Build history of the part. All positions in model axes, mm. Face numbers are marked on the shaded views. A direction names the side the tool comes from. Round coordinates to 2 decimals unless told otherwise and drop trailing zeros. Order: outer loops, then holes, each group sorted by start corner. A loop starts at its lowest first (then second) coordinate and runs counter-clockwise, first axis right, second up. Notation, with made-up numbers: M 70,37 L 109,37 A19 cw 109,57 Z; hole C 66.25,-27 d8. An arc over 180 degrees is marked long. One line per item, written item: value. Start each with the question number.
Item 1: Pin check, flat tips, straight feed: pin 1 (4 mm diameter, centred on y = 52, z = 318.5, fed in from -X); pin 2 (17 mm diameter, centred on x = -101.5, y = 0, fed in from +Z); pin 3 (3 mm diameter, centred on y = 176.5, z = 327, fed in from -X). Stop position of each tip, or through.
Item 2: Band-saw the part on B-B, the plane y = 56.5. Write the cut outline in (x, z).
Item 3: Band-saw the part on C-C, the plane z = 386. Write the cut outline in (x, y).
Item 4: Tool access for the marked faces 1, 2 and 3: list every direction of +Z, -Z, +X, -X, +Y, -Y with a clear straight run to the whole face (end or side of a thin tool).
Item 5: Band-saw the part on A-A, the plane z = 174.5. Write the cut outline in (x, y), then the cut area to 3 significant figures.
Item 6: Band-saw the part on D-D, the plane x = -101.5. Write the cut outline in (y, z).
Item 7: Probe L1, parallel to X at y = 205, z = 174.5; L2, parallel to Y at x = 101.5, z = 150.5; L3, parallel to Y at x = 77.5, z = 200.5. List the from-to ranges inside material, lowest first.
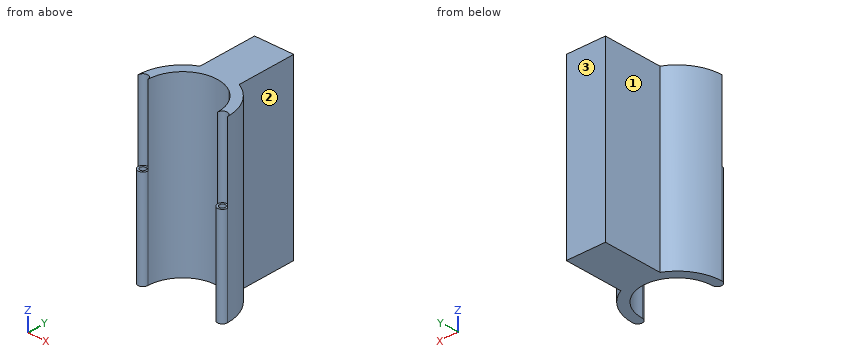
```python
from build123d import *

# Parameters (mm, degrees)
BOSS_EXTRU_1_DEPTH      = 450
ESQUISSE2_R             = 7.5
ENL_V_MAT_EXTRU_1_DEPTH = 350
ESQUISSE2_3_R           = 12.5
ESQUISSE2_3_R_2         = 7.5
ENL_V_MAT_EXTRU_2_DEPTH = 200


with BuildPart() as part:
    # Esquisse1 → Boss.-Extru.1 (new body)
    with BuildSketch(Plane.XY):
        with BuildLine():
            Line((-50, 253.627440537), (-50, 102.449987799))
            ThreePointArc((-50, 102.449987799), (0, 114), (50, 102.449987799))
            Line((50, 102.449987799), (50, 253.627440537))
            Line((50, 253.627440537), (-50, 253.627440537))
        make_face()
        with BuildLine():
            ThreePointArc((-89, 0), (-78.647949751, 41.659332688), (-50, 73.627440537))
            Line((-50, 73.627440537), (-50, 102.449987799))
            ThreePointArc((-50, 102.449987799), (-96.685055722, 60.398675482), (-114, 0))
            ThreePointArc((-114, 0), (-101.5, -12.5), (-89, 0))
        make_face()
        with BuildLine():
            Line((-50, 102.449987799), (-50, 73.627440537))
            ThreePointArc((-50, 73.627440537), (0, 89), (50, 73.627440537))
            Line((50, 73.627440537), (50, 102.449987799))
            ThreePointArc((50, 102.449987799), (0, 114), (-50, 102.449987799))
        make_face()
        with BuildLine():
            Line((50, 102.449987799), (50, 73.627440537))
            ThreePointArc((50, 73.627440537), (78.647949751, 41.659332688), (89, 0))
            ThreePointArc((89, 0), (101.5, -12.5), (114, 0))
            ThreePointArc((114, 0), (96.685055722, 60.398675482), (50, 102.449987799))
        make_face()
    extrude(amount=BOSS_EXTRU_1_DEPTH)

    # Esquisse2 → Enl_v. mat.-Extru.1 (cut)
    with BuildSketch(Plane.XY.offset(450)):
        with Locations((101.5, 0)):
            Circle(ESQUISSE2_R)
        with Locations((-101.5, 0)):
            Circle(ESQUISSE2_R)
    extrude(amount=-ENL_V_MAT_EXTRU_1_DEPTH, mode=Mode.SUBTRACT)

    # Esquisse2_3 → Enl_v. mat.-Extru.2 (cut)
    # profile 1 of 2: a face of its own
    with BuildSketch(Plane.XY.offset(450)):
        with Locations((-101.5, 0)):
            Circle(ESQUISSE2_3_R)
        with Locations((-101.5, 0)):
            Circle(ESQUISSE2_3_R_2, mode=Mode.SUBTRACT)
    # profile 2 of 2: a face of its own
    with BuildSketch(Plane.XY.offset(450)):
        with Locations((101.5, 0)):
            Circle(ESQUISSE2_3_R)
        with Locations((101.5, 0)):
            Circle(ESQUISSE2_3_R_2, mode=Mode.SUBTRACT)
    extrude(amount=-ENL_V_MAT_EXTRU_2_DEPTH, mode=Mode.SUBTRACT)


solid = part.part
```
Output:
1. pin 1: stops at x = -102.45
1. pin 2: stops at z = 250
1. pin 3: stops at x = -50
2. outline: M -99.01,0 L -68.77,0 L -68.77,450 L -99.01,450 Z; M 68.77,0 L 99.01,0 L 99.01,450 L 68.77,450 Z
3. outline: M -114,0 A12.5 cw -89,0 A89 cw 89,0 A12.5 cw 114,0 A114 ccw 50,102.45 L 50,253.63 L -50,253.63 L -50,102.45 A114 ccw Z
4. face 1: +Z, -Z, -X, +Y
4. face 2: +Z, -Z, +X, +Y
4. face 3: +Z, -Z, +X, -X, +Y
5. outline: M -114,0 A12.5 ccw -89,0 A89 cw 89,0 A12.5 ccw 114,0 A114 ccw 50,102.45 L 50,253.63 L -50,253.63 L -50,102.45 A114 ccw Z; hole C -101.5,0 d15; hole C 101.5,0 d15
5. area: 22,400 mm²
6. outline: M -12.5,0 L 51.9,0 L 51.9,450 L 12.5,450 L 12.5,250 L 7.5,250 L 7.5,100 L -7.5,100 L -7.5,250 L -12.5,250 Z
7. L1: x = -50 to 50
7. L2: y = -12.5 to -7.5, 7.5 to 51.9
7. L3: y = 43.76 to 83.6
